Answer from the drawing. Dimensions are ordinates in mm from the lowest x, y and z of the part. A direction names the side the tool comes from. Coordinates: 2 decimals unless noted, no trailing zeros. Loops run counter-clockwise (first coordinate to the right, second up) from the corner with the lowest first, then second, coordinate; pieces in that order, holes last. Notation, with made-up numbers: (36, 86) -> (95, 86) arc R14 cw to (95, 93) -> close; hole circle Ø5 at (20, -17.75). An arc over 180 degrees is marked (long way). Use a Markdown table: item, result.
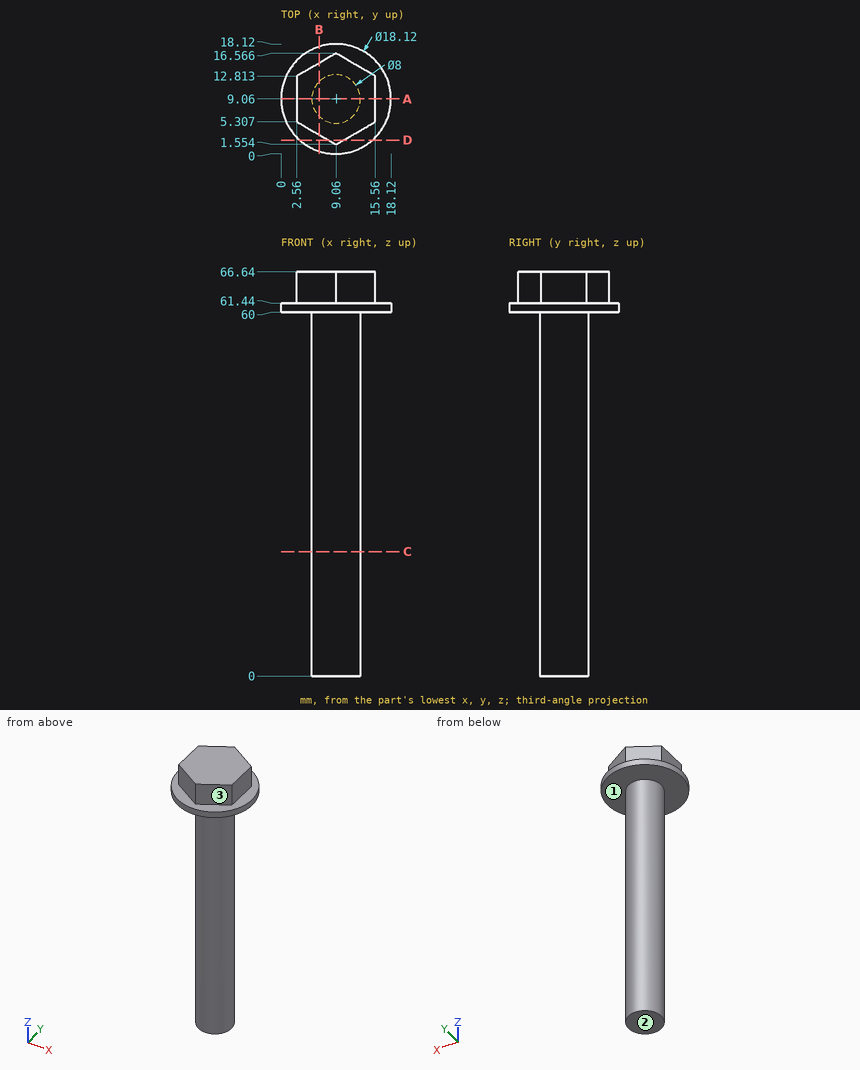
Q1. Section D-D on y = 2.25 is taken. Determine the outline of the cut face in (x, z) (1 decimal).
Solved:
| item | result |
|---|---|
| outline | (3.1, 60) -> (15, 60) -> (15, 61.4) -> (10.3, 61.4) -> (10.3, 66.6) -> (7.9, 66.6) -> (7.9, 61.4) -> (3.1, 61.4) -> close |
Q2. Section C-C on z = 20.5 is taken. Determine the outline of the cut face in (x, y).
Solved:
| item | result |
|---|---|
| outline | circle Ø8 at (9.06, 9.06) |
Q3. Consider line 1 (Z direction, x = 15, y = 7.75); line 2 (X direction, y = 10.5, z = 64.5); line 3 (Z direction, x = 1.5, y = 6.5). Determine where each line is inside the solid, lowest interval first. Write a range as [from, to].
Solved:
| item | result |
|---|---|
| line 1 | [60, 66.64] |
| line 2 | [2.56, 15.56] |
| line 3 | [60, 61.44] |
Q4. Given pin 1 Ø6 at (y, z) = (13.5, 14) entering from -X; pin 2 Ø4 at (x, z) = (13, 14.5) entering from +Y; pin 3 Ø10 at (x, z) = (7.5, 19.5) entering from +Y, each flat-ended and moving along its own axis, determine where each tip first touches the part or whether it passes through.
Solved:
| item | result |
|---|---|
| pin 1 | x = 5.33 |
| pin 2 | y = 12.56 |
| pin 3 | y = 13.06 |
Q5. Section A-A on y = 9.06 is taken. Determine the outline of the cut face in (x, z).
Solved:
| item | result |
|---|---|
| outline | (0, 60) -> (5.06, 60) -> (5.06, 0) -> (13.06, 0) -> (13.06, 60) -> (18.12, 60) -> (18.12, 61.44) -> (15.56, 61.44) -> (15.56, 66.64) -> (2.56, 66.64) -> (2.56, 61.44) -> (0, 61.44) -> close |
Q6. For the marked faces 1, 2 and 3, determine the directions among +Z, -Z, +X, -X, +Y, -Y from which every point of the face is accessible in a straight line to the end or side of a thin tool.
Solved:
| item | result |
|---|---|
| face 1 | -Z |
| face 2 | -Z, +X, -X, +Y, -Y |
| face 3 | +Z, +X, -Y |
Q7. Section B-B on x = 6.25 is taken. Determine the outline of the cut face in (y, z).
Solved:
| item | result |
|---|---|
| outline | (0.45, 60) -> (6.21, 60) -> (6.21, 0) -> (11.91, 0) -> (11.91, 60) -> (17.67, 60) -> (17.67, 61.44) -> (14.94, 61.44) -> (14.94, 66.64) -> (3.18, 66.64) -> (3.18, 61.44) -> (0.45, 61.44) -> close |
